```python
from build123d import *

# Parameters (mm, degrees)
SKETCH1_R          = 5
BASE_EXTRUDE_DEPTH = 5


with BuildPart() as part:
    # Sketch1 → Base-Extrude (new, symmetric)
    with BuildSketch(Plane.XY):
        with BuildLine():
            Line((9.397696336, 105.05059331), (78.039168607, -22.671373759))
            ThreePointArc((78.039168607, -22.671373759), (78.813241725, -30.264373144), (74.00519187, -36.191892476))
            ThreePointArc((74.00519187, -36.191892476), (-2.017468863, -54.986869829), (-77.525144227, -34.21941742))
            ThreePointArc((-77.525144227, -34.21941742), (-82.177273716, -28.168754641), (-81.205819752, -20.598476837))
            Line((-81.205819752, -20.598476837), (-9.263046944, 105.293500781))
            ThreePointArc((-9.263046944, 105.293500781), (0.138865491, 110.667985076), (9.397696336, 105.05059331))
        make_face()
        with Locations((0, -40)):
            Circle(SKETCH1_R, mode=Mode.SUBTRACT)
        with Locations((0, 100)):
            Circle(SKETCH1_R, mode=Mode.SUBTRACT)
    extrude(amount=BASE_EXTRUDE_DEPTH, both=True)


solid = part.part
```
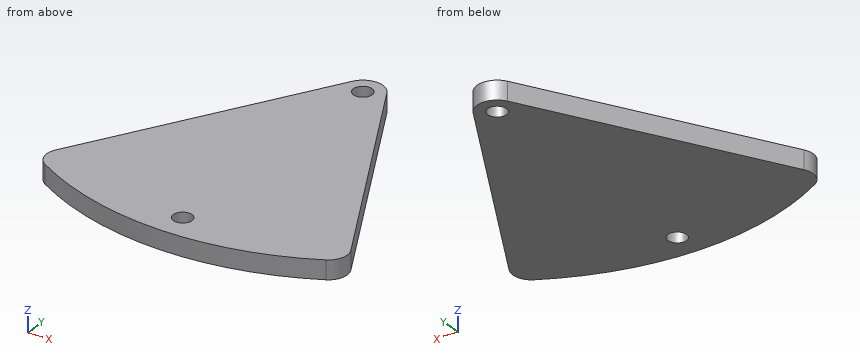
For this review, take the finished solid that the model builds, in its own axes (mm). Round coordinates to 2 decimals unless told otherwise and drop trailing zeros. Loops run counter-clockwise (first coordinate to the right, second up) from the corner with the lowest first, then second, coordinate; pieces in that order, holes last.
Q1. Insertion check: pin 1 Ø13 at (x, y) = (0, -40) entering from -Z; pin 2 Ø5 at (y, z) = (59, 4) entering from +X; pin 3 Ø3 at (y, z) = (44, 1.5) entering from -X; pin 4 Ø4 at (x, z) = (-30, 1.5) entering from +Y. Each pin has a flat end and moves straight along its axis. Give the tip position at first contact, or say it passes through.
Result sheet:
pin 1: stops at z = -5
pin 2: stops at x = 35.49
pin 3: stops at x = -45.15
pin 4: stops at y = 72.51
Q2. Add section D-D on y = -40. Write out the cut boundary in (x, z).
Result sheet:
outline: (-66.52, -5) - (-5, -5) - (-5, 5) - (-66.52, 5) - close; (5, -5) - (66.52, -5) - (66.52, 5) - (5, 5) - close
Q3. Add section A-A on x = 0. Write out the cut boundary in (y, z), plus the area to 3 significant figures.
Result sheet:
outline: (-55, -5) - (-45, -5) - (-45, 5) - (-55, 5) - close; (-35, -5) - (95, -5) - (95, 5) - (-35, 5) - close; (105, -5) - (110.67, -5) - (110.67, 5) - (105, 5) - close
area: 1,460 mm2
Q4. Add section B-B on z = 3.25. Write out the cut boundary in (x, y).
Result sheet:
outline: (-81.21, -20.6) arc R10 ccw to (-77.53, -34.22) arc R155 ccw to (74.01, -36.19) arc R10 ccw to (78.04, -22.67) - (9.4, 105.05) arc R10.67 ccw to (-9.26, 105.29) - close; hole circle Ø10 at (0, -40); hole circle Ø10 at (0, 100)
Q5. To check wall thickness, follow line 1 along Y through (x, z) = (0, 0.75); line 2 along Y through (x, z) = (-2, 3.5); line 3 along X through (y, z) = (-35.5, -1.5). State the ranges of each line that lie inside material, in increasing order.
Result sheet:
line 1: y = -55 to -45, -35 to 95, 105 to 110.67
line 2: y = -54.99 to -44.58, -35.42 to 95.42, 104.58 to 110.48
line 3: x = -75.26 to -2.18, 2.18 to 75.1
Q6. Add section C-C on y = 100. Write out the cut boundary in (x, z).
Result sheet:
outline: (-12.29, -5) - (-5, -5) - (-5, 5) - (-12.29, 5) - close; (5, -5) - (12.11, -5) - (12.11, 5) - (5, 5) - close
